Verification items for the finished model (mm, model axes). Round coordinates to 2 decimals unless told otherwise and drop trailing zeros. Write each loop counter-clockwise with the first axis right and the second up, starting at its lowest first coordinate (ties: lowest second). Pieces come first, ordered by that corner, then holes. Notation, with made-up numbers: (64.25, 24) - (112.25, 24) arc R27 ccw to (112.25, 44) - close; hole circle Ø8 at (-31.75, -36). An arc over 180 degrees is marked (long way). Answer as a JSON object with one key per item and string values.
```python
from build123d import *

# Parameters (mm, degrees)
SKETCH1_W          = 50
SKETCH1_H          = 83.414309181
BASE_FLANGE1_DEPTH = 1.3
FILLET1_R          = 5
SKETCH6_R          = 9.5
CUT_EXTRUDE1_DEPTH = 10
SKETCH7_R          = 2.25
CUT_EXTRUDE2_DEPTH = 10


# Sheet-metal steps are written as plain solids
with BuildPart() as part:
    # Sketch1 → Base-Flange1 (new body)
    with BuildSketch(Plane(origin=(0, 0, 0), x_dir=(1, 0, 0), z_dir=(0, 1, 0))):
        with Locations((-0.387063477, 0.292845409)):
            Rectangle(SKETCH1_W, SKETCH1_H)
    extrude(amount=-BASE_FLANGE1_DEPTH)

    # Fillet1
    fillet1_edges = [part.edges().sort_by_distance(p)[0] for p in [
        (24.612936523, -0.65, 41.414309181),
        (-25.387063477, -0.65, 41.414309181),
        (-25.387063477, -0.65, -42),
        (24.612936523, -0.65, -42),
    ]]
    fillet(fillet1_edges, radius=FILLET1_R)

    # Sketch6 → Cut-Extrude1 (cut)
    with BuildSketch(Plane(origin=(0, 0, 0), x_dir=(1, 0, 0), z_dir=(0, 1, 0))):
        with Locations(Location((0, 22, 0), (0, 0, 270))):
            Circle(SKETCH6_R)
        with Locations(Location((0, -21.414309181, 0), (0, 0, 270))):
            Circle(SKETCH6_R)
    extrude(amount=-CUT_EXTRUDE1_DEPTH, mode=Mode.SUBTRACT)

    # Sketch7 → Cut-Extrude2 (cut)
    with BuildSketch(Plane(origin=(0, 0, 0), x_dir=(1, 0, 0), z_dir=(0, 1, 0))):
        with Locations(Location((19.612936523, 37, 0), (0, 0, 270))):
            Circle(SKETCH7_R)
        with Locations(Location((-20.387063477, 37, 0), (0, 0, 270))):
            Circle(SKETCH7_R)
        with Locations(Location((-20.387063477, -36.414309181, 0), (0, 0, 270))):
            Circle(SKETCH7_R)
        with Locations(Location((19.612936523, -36.414309181, 0), (0, 0, 270))):
            Circle(SKETCH7_R)
    extrude(amount=-CUT_EXTRUDE2_DEPTH, mode=Mode.SUBTRACT)


solid = part.part
```
1. Cross-section at D-D (z = 14). Record the boundary of the cut face in (x, y), plus the area to 3 significant figures.
Completed:
{"outline": "(-25.39, -1.3) - (-5.94, -1.3) - (-5.94, 0) - (-25.39, 0) - close; (5.94, -1.3) - (24.61, -1.3) - (24.61, 0) - (5.94, 0) - close", "area": "49.6 mm^2"}
2. Go/stop test with a flat-tipped pin: pin 1 (3 mm diameter, centred on x = -13.5, z = 3.5, fed in from +Y). Record where the tip stops, or that it passes through.
Completed:
{"pin 1": "stops at y = 0"}
3. Cross-section at C-C (y = -0.55). Record the boundary of the cut face in (x, z), plus the area to 3 significant figures.
Completed:
{"outline": "(-25.39, -37) arc R5 ccw to (-20.39, -42) - (19.61, -42) arc R5 ccw to (24.61, -37) - (24.61, 36.41) arc R5 ccw to (19.61, 41.41) - (-20.39, 41.41) arc R5 ccw to (-25.39, 36.41) - close; hole circle Ø4.5 at (-20.39, -37); hole circle Ø4.5 at (-20.39, 36.41); hole circle Ø19 at (0, -22); hole circle Ø19 at (0, 21.41); hole circle Ø4.5 at (19.61, -37); hole circle Ø4.5 at (19.61, 36.41)", "area": "3,520 mm^2"}
4. Mould release check, pull along X, two halves, no side actions. Record for faces 1 (the face through (-1, 0, -1)), 2 (the face through (-23.96, -0.66, -40.5)), 3 (the face through (20.29, -0.64, 38.56)): released by +X, released by -X, zero draft, split by the parting line, or undercut.
Completed:
{"face 1": "zero draft", "face 2": "released by -X", "face 3": "undercut"}
5. Cross-section at B-B (x = 0). Record the boundary of the cut face in (y, z).
Completed:
{"outline": "(-1.3, -42) - (0, -42) - (0, -31.5) - (-1.3, -31.5) - close; (-1.3, -12.5) - (0, -12.5) - (0, 11.91) - (-1.3, 11.91) - close; (-1.3, 30.91) - (0, 30.91) - (0, 41.41) - (-1.3, 41.41) - close"}
6. Cross-section at A-A (z = -22). Record the boundary of the cut face in (x, y).
Completed:
{"outline": "(-25.39, -1.3) - (-9.5, -1.3) - (-9.5, 0) - (-25.39, 0) - close; (9.5, -1.3) - (24.61, -1.3) - (24.61, 0) - (9.5, 0) - close"}
7. Material ranges on probe 1 along Z at (x, y) = (19, -0.55); probe 2 along Z at (x, y) = (-4.5, -0.35); probe 3 along X at (y, z) = (-0.1, 19), recorded low to high. Write a range as from..to.
Completed:
{"probe 1": "z = -42..-39.16, -34.84..34.25, 38.58..41.41", "probe 2": "z = -42..-30.37, -13.63..13.05, 29.78..41.41", "probe 3": "x = -25.39..-9.19, 9.19..24.61"}
